from build123d import *

# Parameters (mm, degrees)
SKETCH_1_W          = 23.1
SKETCH_1_H          = 4.6
SKETCH_1_H_2        = 2.4
SKETCH_1_W_2        = 4.75
SKETCH_1_H_3        = 16.5
EXTRUDE_1_DEPTH     = 12.3
SKETCH_2_R          = 5.75
SKETCH_2_R_2        = 2.8
EXTRUDE_3_DEPTH     = 4.2
SKETCH_4_R          = 2.5
EXTRUDE_4_DEPTH     = 4.2
SKETCH_5_W          = 4.7
SKETCH_5_H          = 2.5
EXTRUDE_5_DEPTH     = 8
SKETCH_6_W          = 4.7
SKETCH_6_H          = 2.5
EXTRUDE_6_DEPTH     = 5
SKETCH_7_R          = 0.965
CUT_EXTRUDE_1_DEPTH = 7


with BuildPart() as part:
    # 草图1 → 凸台-拉伸1 (new body)
    with BuildSketch(Plane.XY):
        with Locations((0, 9.45)):
            Rectangle(SKETCH_1_W, SKETCH_1_H)
        with Locations((0, 5.95)):
            Rectangle(SKETCH_1_W, SKETCH_1_H_2)
        with Locations((-13.925, 5.95)):
            Rectangle(SKETCH_1_W_2, SKETCH_1_H_2)
        with Locations((13.925, 5.95)):
            Rectangle(SKETCH_1_W_2, SKETCH_1_H_2)
        with Locations((0, -3.5)):
            Rectangle(SKETCH_1_W, SKETCH_1_H_3)
    extrude(amount=EXTRUDE_1_DEPTH)

    # 草图2 → 凸台-拉伸3 (add)
    with BuildSketch(Plane(origin=(0, 11.75, 0), x_dir=(1, 0, 0), z_dir=(0, 1, 0))):
        with Locations((5.4, -6.15)):
            Circle(SKETCH_2_R)
        with Locations((-0.65, -6.15)):
            Circle(SKETCH_2_R_2)
        with Locations((-0.65, -6.15)):
            Circle(SKETCH_2_R_2)
        with Locations((5.4, -6.15)):
            Circle(SKETCH_2_R)
        with Locations((5.4, -6.15)):
            Circle(SKETCH_2_R)
        with Locations((-0.65, -6.15)):
            Circle(SKETCH_2_R_2)
    extrude(amount=EXTRUDE_3_DEPTH)

    # 草图4 → 凸台-拉伸4 (add)
    with BuildSketch(Plane(origin=(0, 15.95, 0), x_dir=(1, 0, 0), z_dir=(0, 1, 0))):
        with Locations(Location((5.4, -6.15, 0), (0, 0, 270))):
            Circle(SKETCH_4_R)
    extrude(amount=EXTRUDE_4_DEPTH)

    # 草图5 → 凸台-拉伸5 (add)
    with BuildSketch(Plane(origin=(11.55, 0, 0), x_dir=(0, 0, -1), z_dir=(1, 0, 0))):
        with Locations((-6.15, -6.5)):
            Rectangle(SKETCH_5_W, SKETCH_5_H)
    extrude(amount=EXTRUDE_5_DEPTH)

    # 草图6 → 凸台-拉伸6 (add)
    with BuildSketch(Plane(origin=(19.55, 0, 0), x_dir=(0, 0, -1), z_dir=(1, 0, 0))):
        with Locations((-6.15, -6.5)):
            Rectangle(SKETCH_6_W, SKETCH_6_H)
    extrude(amount=EXTRUDE_6_DEPTH)

    # 草图7 → 切除-拉伸1 (cut)
    with BuildSketch(Plane(origin=(0, 7.15, 0), x_dir=(1, 0, 0), z_dir=(0, 1, 0))):
        with Locations(Location((-13.925, -6.15, 0), (0, 0, 180))):
            Circle(SKETCH_7_R)
    extrude(amount=-CUT_EXTRUDE_1_DEPTH, mode=Mode.SUBTRACT)


solid = part.part
Read the model definition and answer for the solid it produces. Units are mm, in the model's axes. A direction names the side the tool comes from. Round coordinates to 2 decimals unless told otherwise and drop trailing zeros. Write each loop counter-clockwise with the first axis right and the second up, starting at its lowest first coordinate (ties: lowest second). Pieces come first, ordered by that corner, then holes.
1. Given pin 1 Ø2.5 at (x, z) = (14, 7.5) entering from +Y; pin 2 Ø12 at (x, y) = (14, 15.5) entering from +Z; pin 3 Ø5 at (x, z) = (21, 5.5) entering from +Y; pin 4 Ø0.8 at (x, y) = (15.5, -6.5) entering from +Z, each flat-ended and moving along its own axis, determine where each tip first touches the part or whether it passes through.
2. Straight lines are drawn through the part: L1, parallel to Y at x = 14, z = 4; L2, parallel to Y at x = -4.5, z = 2.5; L3, parallel to Y at x = -3, z = 5. For each, find the intervals that lie inside material, in ascending order.
3. Which of the six approach directions +Z, -Z, +X, -X, +Y, -Y give full straight-line access (tool end or side, diameter ignored) to faces 1 (the face through (-11.55, 9, 6)), 2 (the face through (-5, 11.75, 6)), 3 (the face through (-14, 4.75, 7.4))?
4. The part is cut by section D-D, the plane y = 3. Determine the outline of the cut face in (x, z), then the cut area to 3 significant figures.
5. The part is cut by section B-B, the plane x = 13. Determine the outline of the cut face in (y, z), then the cut area to 3 significant figures.
6. The part is cut by section C-C, the plane x = -0.65. Determine the outline of the cut face in (y, z), then the cut area to 3 significant figures.
7. Determine the mould class of faces 4 (the face through (18, -7, 8.5)), 5 (the face through (2.96, 18.02, 5.61)), 6 (the face through (11.55, 9, 6)), 7 (the face through (-12.96, 5.97, 6.19)) for opening direction Z: pulls with the +Z half, pulls with the -Z half, needs draft (parallel to the pull), parting line crosses it, or undercut.
8. The part is cut by section A-A, the plane z = 6.15. Determine the outline of the cut face in (x, y).
Values:
1. pin 1: stops at y = 7.15
1. pin 2: stops at z = 12.3
1. pin 3: stops at y = -5.25
1. pin 4: stops at z = 8.5
2. L1: y = -7.75 to -5.25, 4.75 to 7.15
2. L2: y = -11.75 to 11.75
2. L3: y = -11.75 to 15.95
3. face 1: +Z, -Z, -X, +Y
3. face 2: +Y
3. face 3: +Z, -Z, -X, -Y
4. outline: (-11.55, 0) - (11.55, 0) - (11.55, 12.3) - (-11.55, 12.3) - close
4. area: 284 mm2
5. outline: (-7.75, 3.8) - (-5.25, 3.8) - (-5.25, 8.5) - (-7.75, 8.5) - close; (4.75, 0) - (7.15, 0) - (7.15, 12.3) - (4.75, 12.3) - close
5. area: 41.3 mm2
6. outline: (-11.75, 0) - (11.75, 0) - (11.75, 3.35) - (15.95, 3.35) - (15.95, 8.95) - (11.75, 8.95) - (11.75, 12.3) - (-11.75, 12.3) - close
6. area: 313 mm2
7. face 4: pulls with the +Z half
7. face 5: parting line crosses it
7. face 6: needs draft
7. face 7: undercut
8. outline: (-16.3, 4.75) - (-14.89, 4.75) - (-14.89, 7.15) - (-16.3, 7.15) - close; (-12.96, 4.75) - (-11.55, 4.75) - (-11.55, -11.75) - (11.55, -11.75) - (11.55, -7.75) - (24.55, -7.75) - (24.55, -5.25) - (11.55, -5.25) - (11.55, 4.75) - (16.3, 4.75) - (16.3, 7.15) - (11.55, 7.15) - (11.55, 11.75) - (11.15, 11.75) - (11.15, 15.95) - (7.9, 15.95) - (7.9, 20.15) - (2.9, 20.15) - (2.9, 15.95) - (-3.45, 15.95) - (-3.45, 11.75) - (-11.55, 11.75) - (-11.55, 7.15) - (-12.96, 7.15) - close
